Could you check a few things on this model? Use its own coordinates, in mm. Coordinates: 2 decimals unless noted, no trailing zeros. Loops run counter-clockwise (first coordinate to the right, second up) from the corner with the lowest first, then second, coordinate; pieces in that order, holes last.
Autodesk Fusion 360 part; units mm, degrees
sketch "スケッチ1" plane through (0, 0, 0) normal (0, 1, 0) x (1, 0, 0)
  line L0 (-10.375, 2) -> (10.375, 2)
  line L1 (10.375, 2) -> (10.375, -64)
  line L2 (10.375, -64) -> (-10.375, -64)
  line L3 (-10.375, -64) -> (-10.375, 2)
  line L4 (0, 0) -> (0, -64)
  circle A0 centre (7.5, -8) radius 1.1
  circle A1 centre (7.5, -8) radius 1.85
  circle A2 centre (7.5, -60.5) radius 1.1
  circle A3 centre (7.5, -60.5) radius 1.85
  line L5 (-10.375, -2) -> (10.375, -2)
  circle A4 centre (-7.5, -8) radius 1.85
  circle A5 centre (-7.5, -8) radius 1.1
  circle A6 centre (-7.5, -60.5) radius 1.85
  circle A7 centre (-7.5, -60.5) radius 1.1
  circle A8 centre (-6, -44.5) radius 1.1
  circle A9 centre (-6, -44.5) radius 1.85
  dimension "d1" = 66
  dimension "d2" = 20.75
  dimension "d3" = 10.375
  dimension "d4" = 2.2
  dimension "d6" = 10
  dimension "d7" = 3.7
  dimension "d8" = 2.2
  dimension "d9" = 3.7
  dimension "d11" = 62.5
  dimension "d12" = 7.5
  dimension "d13" = 7.5
  dimension "d14" = 4
  dimension "d27" = 3.7
  dimension "d28" = 2.2
  dimension "d29" = 6
  dimension "d30" = 46.5
extrude "押し出し4" add sketch "スケッチ1" along normal blind 0.7 contours L0 L1 L3 L5 | L2 L3 L4 L5 | L1 L2 L4 L5 | A1 | A3 | A4 | A6 | A8 | A9 makes body 1
extrude "押し出し5" add sketch "スケッチ1" along normal blind 2.4 separate body contours L2 L3 L4 L5 | L1 L2 L4 L5 | A1 | A3 | A4 | A6 | A8 | A9 makes body 2
combine "結合1" operation add target body 2 tool bodies 1
extrude "押し出し6" cut sketch "スケッチ1" along normal blind 1.4 contours A1 | A3 | A4 | A6 bodies 2
extrude "押し出し7" cut sketch "スケッチ1" along normal blind 2.4 contours A8 bodies 2
extrude "押し出し8" cut sketch "スケッチ1" along normal blind 1.4 contours A9 bodies 2
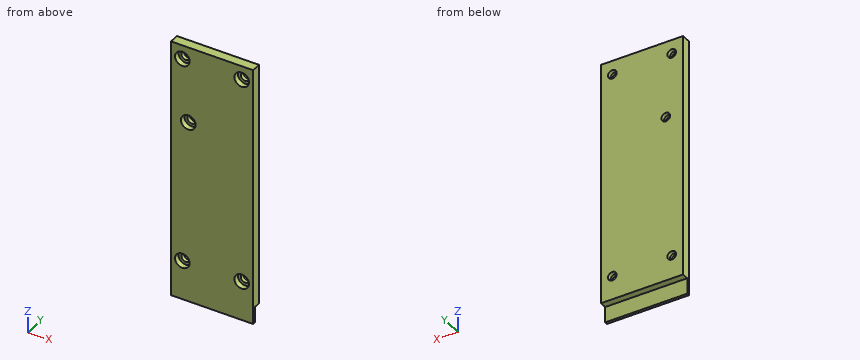
(1) Imagine slicing it at C-C, the plane y = 1.9. Write out the boundary of the cut face in (x, z) (3 decimals).
Answers:
outline: (-10.375, 2) - (10.375, 2) - (10.375, 64) - (-10.375, 64) - close; hole circle Ø2.2 at (-7.5, 8); hole circle Ø2.2 at (-7.5, 60.5); hole circle Ø2.2 at (-6, 44.5); hole circle Ø2.2 at (7.5, 8); hole circle Ø2.2 at (7.5, 60.5)
(2) Imagine slicing it at A-A, the plane z = 44.5. Write out the boundary of the cut face in (x, y) (3 decimals).
Answers:
outline: (-10.375, 0) - (-7.85, 0) - (-7.85, 1.4) - (-7.1, 1.4) - (-7.1, 2.4) - (-10.375, 2.4) - close; (-4.9, 1.4) - (-4.15, 1.4) - (-4.15, 0) - (10.375, 0) - (10.375, 2.4) - (-4.9, 2.4) - close
(3) Imagine slicing it at B-B, the plane x = 7.5. Write out the boundary of the cut face in (y, z), and give its area (3 significant figures).
Answers:
outline: (0, -2) - (0.7, -2) - (0.7, 2) - (2.4, 2) - (2.4, 6.9) - (1.4, 6.9) - (1.4, 6.15) - (0, 6.15) - close; (0, 9.85) - (1.4, 9.85) - (1.4, 9.1) - (2.4, 9.1) - (2.4, 59.4) - (1.4, 59.4) - (1.4, 58.65) - (0, 58.65) - close; (0, 62.35) - (1.4, 62.35) - (1.4, 61.6) - (2.4, 61.6) - (2.4, 64) - (0, 64) - close
area: 137 mm2
(4) I need wall thicknesses on probe 1 along X at (y, z) = (0.5, 8) (3 decimals); probe 2 along X at (y, z) = (1.65, 8) (3 decimals); probe 3 along Z at (x, y) = (7.5, 2). Which ranges of each line are inside material? Lowest first, please.
Answers:
probe 1: x = -10.375 to -9.35, -5.65 to 5.65, 9.35 to 10.375
probe 2: x = -10.375 to -8.6, -6.4 to 6.4, 8.6 to 10.375
probe 3: z = 2 to 6.9, 9.1 to 59.4, 61.6 to 64
(5) Imagine slicing it at D-D, the plane z = 60.5. Write out the boundary of the cut face in (x, y) (3 decimals).
Answers:
outline: (-10.375, 0) - (-9.35, 0) - (-9.35, 1.4) - (-8.6, 1.4) - (-8.6, 2.4) - (-10.375, 2.4) - close; (-6.4, 1.4) - (-5.65, 1.4) - (-5.65, 0) - (5.65, 0) - (5.65, 1.4) - (6.4, 1.4) - (6.4, 2.4) - (-6.4, 2.4) - close; (8.6, 1.4) - (9.35, 1.4) - (9.35, 0) - (10.375, 0) - (10.375, 2.4) - (8.6, 2.4) - close
(6) For pin 1 (1.8 mm diameter, centred on x = -6, z = 44.5, fed in from +Y); pin 2 (3 mm diameter, centred on x = -7.5, z = 60.5, fed in from -Y); pin 3 (0.5 mm diameter, centred on x = -4.5, y = 1.5, fed in from -Z), each with a flat end and sliding along its axis, tell me the tip position at first contact or that it passes through.
Answers:
pin 1: passes through
pin 2: stops at y = 1.4
pin 3: stops at z = 2
